Autodesk Inventor part; units mm, degrees
sketch "Эскиз1" plane through (0, 0, 0) normal (0, 1, 0) x (-1, 0, 0)
  arc A0 (294.6508, 19) -> (288.6508, 13) centre (294.6508, 13) ccw
  arc A1 (226.5258, 13) -> (214.5258, 13) centre (220.5258, 13) ccw
  arc A2 (152.4008, 13) -> (140.4008, 13) centre (146.4008, 13) ccw
  arc A3 (4.1508, 13) -> (-1.8492, 19) centre (-1.8492, 13) ccw
  arc A4 (78.2758, 13) -> (66.2758, 13) centre (72.2758, 13) ccw
  arc A5 (294.6508, 83) -> (294.6508, 71) centre (294.6508, 77) ccw
  arc A6 (288.6508, 141) -> (294.6508, 135) centre (294.6508, 141) ccw
  arc A7 (214.5258, 141) -> (226.5258, 141) centre (220.5258, 141) ccw
  arc A8 (140.4008, 141) -> (152.4008, 141) centre (146.4008, 141) ccw
  arc A9 (66.2758, 141) -> (78.2758, 141) centre (72.2758, 141) ccw
  arc A10 (-1.8492, 135) -> (4.1508, 141) centre (-1.8492, 141) ccw
  arc A11 (-1.8492, 71) -> (-1.8492, 83) centre (-1.8492, 77) ccw
  line L0 (-14.8492, 10.5) -> (-14.8492, 143.5)
  line L1 (-14.8492, 10.5) -> (-14.8492, 143.5)
  line L2 (-4.3492, 154) -> (297.1508, 154)
  line L3 (307.6508, 10.5) -> (307.6508, 143.5)
  line L4 (297.1508, 0) -> (-4.3492, 0)
  line L5 (288.6508, 13) -> (226.5258, 13)
  line L6 (214.5258, 13) -> (152.4008, 13)
  line L7 (140.4008, 13) -> (78.2758, 13)
  line L8 (66.2758, 13) -> (4.1508, 13)
  line L9 (-1.8492, 19) -> (-1.8492, 71)
  line L10 (-1.8492, 83) -> (-1.8492, 135)
  line L11 (4.1508, 141) -> (66.2758, 141)
  line L12 (78.2758, 141) -> (140.4008, 141)
  line L13 (152.4008, 141) -> (214.5258, 141)
  line L14 (226.5258, 141) -> (288.6508, 141)
  line L15 (294.6508, 135) -> (294.6508, 83)
  line L16 (294.6508, 71) -> (294.6508, 19)
  line L17 (275.1508, 0) -> (362.1508, 0)
  line L18 (307.6508, 0) -> (-14.8492, 0)
  line L19 (-14.8492, 0) -> (-14.8492, 154)
  line L20 (-14.8492, 154) -> (307.6508, 154)
  line L21 (307.6508, 154) -> (307.6508, 0)
  point P0 (0, 0)
  point P1 (323.6508, -3)
  point P2 (297.1508, 10.5)
  point P3 (-4.3492, 10.5)
  point P4 (-4.3492, 143.5)
  point P5 (146.4008, 13)
  dimension "d0" = 74.125
  dimension "d1" = 74.125
  dimension "d2" = 74.125
  dimension "d3" = 6
  dimension "d4" = 296.5
  dimension "d5" = 322.5
  dimension "d6" = 154
  dimension "d7" = 128
  dimension "d8" = 13
  dimension "d9" = 13
  dimension "d10" = 13
  dimension "d11" = 13
extrude "Выдавливание1" add sketch "Эскиз1" along normal blind 17
extrude "Выдавливание2" add sketch "Эскиз1" along normal blind 5 contours A0 L5 A1 L6 A2 L7 A4 L8 A3 L9 A11 L10 A10 L11 A9 L12 A8 L13 A7 L14 A6 L15 A5 L16 | L0 L19 L20 L2 L21 L3 L17 L4 L18
fillet "Сопряжение1" radius 10.5 4 edges at (-307.6508, 8.5, 0) (14.8492, 8.5, 0) (-307.6508, 8.5, 154) (14.8492, 8.5, 154)
ref_plane "РабПлоскость1" through (0, 14.5, 0) normal (0, 1, 0) x (1, 0, 0)
sketch "Эскиз5" plane through (0, 5, 0) normal (0, 1, 0) x (1, 0, 0)
  line L0 (-140.4008, -13) -> (-78.2758, -13)
  arc A0 (-152.4008, -13) -> (-140.4008, -13) centre (-146.4008, -13) ccw
  line L1 (-214.5258, -13) -> (-152.4008, -13)
  arc A1 (-226.5258, -13) -> (-214.5258, -13) centre (-220.5258, -13) ccw
  line L2 (-288.6508, -13) -> (-226.5258, -13)
  arc A2 (-294.6508, -19) -> (-288.6508, -13) centre (-294.6508, -13) ccw
  line L3 (-294.6508, -71) -> (-294.6508, -19)
  arc A3 (-294.6508, -83) -> (-294.6508, -71) centre (-294.6508, -77) ccw
  line L4 (-294.6508, -135) -> (-294.6508, -83)
  arc A4 (-288.6508, -141) -> (-294.6508, -135) centre (-294.6508, -141) ccw
  line L5 (-226.5258, -141) -> (-288.6508, -141)
  arc A5 (-214.5258, -141) -> (-226.5258, -141) centre (-220.5258, -141) ccw
  line L6 (-152.4008, -141) -> (-214.5258, -141)
  arc A6 (-140.4008, -141) -> (-152.4008, -141) centre (-146.4008, -141) ccw
  line L7 (-78.2758, -141) -> (-140.4008, -141)
  arc A7 (-66.2758, -141) -> (-78.2758, -141) centre (-72.2758, -141) ccw
  line L8 (-4.1508, -141) -> (-66.2758, -141)
  arc A8 (1.8492, -135) -> (-4.1508, -141) centre (1.8492, -141) ccw
  line L9 (1.8492, -83) -> (1.8492, -135)
  arc A9 (1.8492, -71) -> (1.8492, -83) centre (1.8492, -77) ccw
  line L10 (1.8492, -19) -> (1.8492, -71)
  arc A10 (-4.1508, -13) -> (1.8492, -19) centre (1.8492, -13) ccw
  line L11 (-66.2758, -13) -> (-4.1508, -13)
  arc A11 (-78.2758, -13) -> (-66.2758, -13) centre (-72.2758, -13) ccw
  point P0 (0, 0)
sketch "Эскиз4" plane through (0, 14.5, 0) normal (0, 1, 0) x (1, 0, 0)
  line L0 (-140.4008, -13) -> (-78.2758, -13)
  arc A0 (-78.2758, -13) -> (-66.2758, -13) centre (-72.2758, -13) ccw
  line L1 (-66.2758, -13) -> (-4.1508, -13)
  arc A1 (-4.1508, -13) -> (1.8492, -19) centre (1.8492, -13) ccw
  line L2 (1.8492, -19) -> (1.8492, -71)
  arc A2 (1.8492, -71) -> (1.8492, -83) centre (1.8492, -77) ccw
  line L3 (1.8492, -83) -> (1.8492, -135)
  arc A3 (1.8492, -135) -> (-4.1508, -141) centre (1.8492, -141) ccw
  line L4 (-4.1508, -141) -> (-66.2758, -141)
  arc A4 (-66.2758, -141) -> (-78.2758, -141) centre (-72.2758, -141) ccw
  line L5 (-78.2758, -141) -> (-140.4008, -141)
  arc A5 (-140.4008, -141) -> (-152.4008, -141) centre (-146.4008, -141) ccw
  line L6 (-152.4008, -141) -> (-214.5258, -141)
  arc A6 (-214.5258, -141) -> (-226.5258, -141) centre (-220.5258, -141) ccw
  line L7 (-226.5258, -141) -> (-288.6508, -141)
  arc A7 (-288.6508, -141) -> (-294.6508, -135) centre (-294.6508, -141) ccw
  line L8 (-294.6508, -135) -> (-294.6508, -83)
  arc A8 (-294.6508, -83) -> (-294.6508, -71) centre (-294.6508, -77) ccw
  line L9 (-294.6508, -71) -> (-294.6508, -19)
  arc A9 (-294.6508, -19) -> (-288.6508, -13) centre (-294.6508, -13) ccw
  line L10 (-288.6508, -13) -> (-226.5258, -13)
  arc A10 (-226.5258, -13) -> (-214.5258, -13) centre (-220.5258, -13) ccw
  line L11 (-214.5258, -13) -> (-152.4008, -13)
  arc A11 (-152.4008, -13) -> (-140.4008, -13) centre (-146.4008, -13) ccw
  arc A12 (4.3492, -154) -> (14.8492, -143.5) centre (4.3492, -143.5) ccw
  line L12 (14.8492, -143.5) -> (14.8492, -10.5)
  arc A13 (14.8492, -10.5) -> (4.3492, 0) centre (4.3492, -10.5) ccw
  line L13 (4.3492, 0) -> (-297.1508, 0)
  arc A14 (-297.1508, 0) -> (-307.6508, -10.5) centre (-297.1508, -10.5) ccw
  line L14 (-307.6508, -10.5) -> (-307.6508, -143.5)
  arc A15 (-307.6508, -143.5) -> (-297.1508, -154) centre (-297.1508, -143.5) ccw
  line L15 (-297.1508, -154) -> (4.3492, -154)
  arc A16 (-226.5258, -13) -> (-214.5258, -13) centre (-220.5258, -13) ccw
  line L16 (-220.5258, -13) -> (-220.5258, -141)
  line L17 (-146.4008, -13) -> (-146.4008, -141)
  line L18 (-72.2758, -13) -> (-72.2758, -141)
  line L19 (-294.6508, -77) -> (1.8492, -77)
  point P0 (0, 0)
properties part number "Крыша2"
Can you work these out from the model? Positions are in its coordinate system, mm. A direction names the side the tool comes from. Coordinates: 2 decimals unless noted, no trailing zeros. Loops run counter-clockwise (first coordinate to the right, second up) from the corner with the lowest first, then second, coordinate; pieces in that order, holes last. Notation, with made-up numbers: (-22, 37.25) - (9, 37.25) arc R5 cw to (9, 46.25) - close; hole circle Ø1 at (21.5, 10.25). An arc over 180 degrees is marked (long way). Use a Markdown table: item, result.
Item 1: I want a section at C-C on z = 77. Please give me the cut outline in (x, y), and give its area (3 significant figures).
Numbers:
| item | result |
|---|---|
| outline | (-307.65, 0) - (14.85, 0) - (14.85, 17) - (-4.15, 17) - (-4.15, 5) - (-288.65, 5) - (-288.65, 17) - (-307.65, 17) - close |
| area | 2,070 mm2 |
Item 2: We'd pull the mould along Z, two halves only. Please class faces 3 (the face through (-304.5, 8.4, 151)), 4 (the face through (-144, 8, 0)), 5 (the face through (-220.4, 10.9, 19)): released by +Z, released by -Z, zero draft, split by the parting line, or undercut.
Numbers:
| item | result |
|---|---|
| face 3 | released by +Z |
| face 4 | released by -Z |
| face 5 | undercut |
Item 3: For faces 1 (the face through (-304.7, 8.4, 3.2)), 2 (the face through (-290.362, 10.916, 17.196)), which set-ups out of +Z, -Z, +X, -X, +Y, -Y let a thin tool reach every point of the face, with its end or its side?
Numbers:
| item | result |
|---|---|
| face 1 | -Z, -X, +Y, -Y |
| face 2 | +Y |
Item 4: I want a section at B-B on x = -165. Please give me the cut outline in (y, z).
Numbers:
| item | result |
|---|---|
| outline | (0, 0) - (17, 0) - (17, 13) - (5, 13) - (5, 141) - (17, 141) - (17, 154) - (0, 154) - close |
Item 5: If I drill on probe 1 along X at (y, z) = (11.75, 113); probe 2 along Z at (x, y) = (-26, 10.75); probe 3 along X at (y, z) = (10.25, 18), over which ranges is the centre line in solid material (lowest first)? Write a range as from..to.
Numbers:
| item | result |
|---|---|
| probe 1 | x = -307.65..-294.65, 1.85..14.85 |
| probe 2 | z = 0..13, 141..154 |
| probe 3 | x = -307.65..-291.33, -223.84..-217.21, -149.72..-143.08, -75.59..-68.96, -1.47..14.85 |
